Check sheet for the modelled part. Datum: model origin and axes. Units: mm. Face numbers are marked on the shaded views. Round coordinates to 2 decimals unless told otherwise and drop trailing zeros. Write each loop counter-clockwise with the first axis right and the second up, starting at its lowest first coordinate (ties: lowest second). Pieces come first, ordered by that corner, then holes. Notation, with made-up numbers: M 76,-32.75 L 134,-32.75 A27 ccw 134,-16.75 Z; hole C -23,31 d4. An arc over 180 degrees is marked long. Answer in a Markdown table with one row per item.
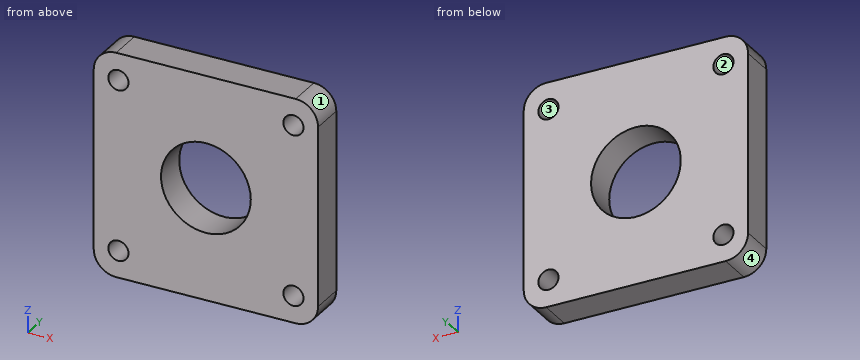
```python
from build123d import *

# Parameters (mm, degrees)
F0_R     = 4.5
F0_R_2   = 20
F1_DEPTH = 15


with BuildPart() as f1:
    # F0 (on Front) → F1 (new body)
    with BuildSketch(Plane.XZ):
        with BuildLine():
            Line((40, 50), (-40, 50))
            ThreePointArc((-40, 50), (-47.071068, 47.071068), (-50, 40))
            Line((-50, 40), (-50, -40))
            ThreePointArc((-50, -40), (-47.071068, -47.071068), (-40, -50))
            Line((-40, -50), (40, -50))
            ThreePointArc((40, -50), (47.071068, -47.071068), (50, -40))
            Line((50, -40), (50, 40))
            ThreePointArc((50, 40), (47.071068, 47.071068), (40, 50))
        make_face()
        with Locations((-39, -38)):
            Circle(F0_R, mode=Mode.SUBTRACT)
        with Locations((39, -38)):
            Circle(F0_R, mode=Mode.SUBTRACT)
        with Locations((-39, 38)):
            Circle(F0_R, mode=Mode.SUBTRACT)
        Circle(F0_R_2, mode=Mode.SUBTRACT)
        with Locations((39, 38)):
            Circle(F0_R, mode=Mode.SUBTRACT)
    extrude(amount=F1_DEPTH)


solid = f1.part
```
1. Draft check along Z on the marked faces 1, 2, 3 and 4. Enter one of: +Z half, -Z half, draft (parallel to the pull), parting line (faces both ways), or undercut.
Found:
| item | result |
|---|---|
| face 1 | +Z half |
| face 2 | undercut |
| face 3 | undercut |
| face 4 | -Z half |
2. Scan lines: L1, parallel to Z at x = -39, y = -7; L2, parallel to Z at x = -40, y = -1; L3, parallel to X at y = -12.75, z = 37. Record each from-to range of solid material in increasing order.
Found:
| item | result |
|---|---|
| L1 | z = -50 to -42.5, -33.5 to 33.5, 42.5 to 50 |
| L2 | z = -50 to -42.39, -33.61 to 33.61, 42.39 to 50 |
| L3 | x = -50 to -43.39, -34.61 to 34.61, 43.39 to 50 |
3. Section check D-D, the plane x = 42. Record the cut outline in (y, z).
Found:
| item | result |
|---|---|
| outline | M -15,-49.8 L 0,-49.8 L 0,-41.35 L -15,-41.35 Z; M -15,-34.65 L 0,-34.65 L 0,34.65 L -15,34.65 Z; M -15,41.35 L 0,41.35 L 0,49.8 L -15,49.8 Z |
4. Section check C-C, the plane z = 38. Record the cut outline in (x, y), and give its area (3 significant figures).
Found:
| item | result |
|---|---|
| outline | M -50,-15 L -43.5,-15 L -43.5,0 L -50,0 Z; M -34.5,-15 L 34.5,-15 L 34.5,0 L -34.5,0 Z; M 43.5,-15 L 50,-15 L 50,0 L 43.5,0 Z |
| area | 1,230 mm2 |
5. Section check B-B, the plane z = 0. Record the cut outline in (x, y), and give its area (3 significant figures).
Found:
| item | result |
|---|---|
| outline | M -50,-15 L -20,-15 L -20,0 L -50,0 Z; M 20,-15 L 50,-15 L 50,0 L 20,0 Z |
| area | 900 mm2 |
6. Section check A-A, the plane y = -10.5. Record the cut outline in (x, z).
Found:
| item | result |
|---|---|
| outline | M -50,-40 A10 ccw -40,-50 L 40,-50 A10 ccw 50,-40 L 50,40 A10 ccw 40,50 L -40,50 A10 ccw -50,40 Z; hole C -39,-38 d9; hole C -39,38 d9; hole C 0,0 d40; hole C 39,-38 d9; hole C 39,38 d9 |
